Read the model definition and answer for the solid it produces. Units are mm, in the model's axes. A direction names the side the tool comes from. Round coordinates to 2 decimals unless told otherwise and drop trailing zeros. Order: outer loops, then holes, each group sorted by start corner. A loop starts at its lowest first (then second) coordinate and runs counter-clockwise, first axis right, second up. Notation, with made-up numbers: (-29.75, 56) -> (-9.75, 56) arc R25 cw to (-9.75, 85) -> close; hole circle Ø2 at (-27, 35). An arc over 180 degrees is marked (long way). One line per item, written item: value. Start each with the question number.
1. For faces 1 (the face through (0, 21, -23.5)), 2 (the face through (0, 13, 23)), 3 (the face through (0, 12, -32)), 4 (the face through (-0.063, 81.182, 64.866)), determine the directions among +Z, -Z, +X, -X, +Y, -Y from which every point of the face is accessible in a straight line to the end or side of a thin tool.
2. Section D-D (z = 10) is taken. Give the vertices of the cut face in (x, y), then the cut area to 3 significant figures.
3. The mould has two halves that part along Y. Classify faces 5 (the face through (0, 9, -37)), 6 (the face through (-11.82, -1.41, 7.9)), 7 (the face through (-0.189, 58.227, 18.773)): released by +Y, released by -Y, zero draft, split by the parting line, or undercut.
4. Section B-B (x = -1.25) is taken. Give the vertices of the cut face in (y, z).
5. Consider line 1 (Y direction, x = -12, z = 30); line 2 (X direction, y = -5, z = 17); line 3 (Z direction, x = -2.75, y = 20.5). Determine where each line is inside the solid, lowest interval first.
6. Section C-C (y = 46.8) is taken. Give the vertices of the cut face in (x, z), then the cut area to 3 significant figures.
7. Flat-ended cylindrical pins translate along their axes: pin 1 Ø5.5 at (y, z) = (-1.5, -30) entering from -X; pin 2 Ø14 at (x, y) = (-4.5, 25) entering from +Z; pin 3 Ø12 at (x, y) = (-4.5, -4.5) entering from +Z; pin 4 Ø2 at (x, y) = (1, 44) entering from -Z. Find the tip coordinate at first contact, or state that the pin passes through.
8. Section A-A (z = -30) is taken. Give the vertices of the cut face in (x, y).
from build123d import *

# Parameters (mm, degrees)
SKETCH1_W           = 27
SKETCH1_H           = 24
BOSS_EXTRUDE1_DEPTH = 37
SHELL1_T            = -3.5
BOSS_EXTRUDE2_DEPTH = 27
SHELL2_START        = -10
SHELL2_DEPTH        = 20
SKETCH3_R           = 2.1
CUT_EXTRUDE1_DEPTH  = 116.92964185
MOVE_FACE1_BY       = 0.1
MOVE_FACE1_2_BY     = 0.1
SKETCH4_R           = 2.1
CUT_EXTRUDE2_DEPTH  = 116.92964185
FILLET1_R           = 5
SKETCH5_W           = 74
SKETCH5_H           = 0.5
CUT_EXTRUDE3_DEPTH  = 116.92964185


# Read off the part's stored shape, not the designer's step: Shell2
with BuildPart() as part:
    # Sketch1 → Boss-Extrude1 (new, symmetric)
    with BuildSketch(Plane.XY):
        Rectangle(SKETCH1_W, SKETCH1_H)
    extrude(amount=BOSS_EXTRUDE1_DEPTH, both=True)

    # Shell1
    shell1_openings = [part.faces().sort_by_distance(p)[0] for p in [
        (0, 0, 37),
        (0, 0, -37),
        (0, -12, 0),
    ]]
    offset(amount=SHELL1_T, openings=shell1_openings, kind=Kind.INTERSECTION)

    # Sketch2 → Boss-Extrude2 (add)
    with BuildSketch(Plane.ZY.offset(13.5)):
        Polygon((63.282032303, 83.924355653), (-27, 31.8), (-27, 12), (21, 12), (21, 31.8), (75.282032303, 63.139745962), align=None)
    extrude(amount=-BOSS_EXTRUDE2_DEPTH)

    # Shell2 outline → Shell2 (cut)
    with BuildSketch(Plane.YZ.offset(SHELL2_START)):
        Polygon((29.779274058, 17.5), (12, 17.5), (12, -23.5), (29.779274058, -23.5), (80.89326674, 65.032032303), (63.139745962, 75.282032303), (31.8, 21), align=None)
    extrude(amount=SHELL2_DEPTH, mode=Mode.SUBTRACT)

    # Sketch3 → Cut-Extrude1 (cut, through all)
    with BuildSketch(Plane.ZY.offset(13.5)):
        with Locations((-30, -1.5)):
            Circle(SKETCH3_R)
        with Locations((-10, -1.5)):
            Circle(SKETCH3_R)
        with Locations((10, -1.5)):
            Circle(SKETCH3_R)
        with Locations((30, -1.5)):
            Circle(SKETCH3_R)
    extrude(amount=-CUT_EXTRUDE1_DEPTH, mode=Mode.SUBTRACT)

    # Move Face1: a face moved inward by 0.1
    extrude(part.faces().sort_by_distance((10, -1.759479058, 0))[0], amount=MOVE_FACE1_BY, dir=(1, 0, 0), mode=Mode.SUBTRACT)

    # Move Face1 2: a face moved inward by 0.1
    extrude(part.faces().sort_by_distance((-10, -1.759479058, 0))[0], amount=MOVE_FACE1_2_BY, dir=(-1, 0, 0), mode=Mode.SUBTRACT)

    # Sketch4 → Cut-Extrude2 (cut, through all)
    with BuildSketch(Plane.ZY.offset(13.5)):
        with Locations((61.621778265, 66.8)):
            Circle(SKETCH4_R)
        with Locations((44.301270189, 56.8)):
            Circle(SKETCH4_R)
        with Locations((26.980762114, 46.8)):
            Circle(SKETCH4_R)
    extrude(amount=-CUT_EXTRUDE2_DEPTH, mode=Mode.SUBTRACT)

    # Fillet1
    fillet1_edges = [part.edges().sort_by_distance(p)[0] for p in [
        (11.75, 31.8, 21),
        (0, 12, 21),
        (-11.75, 31.8, 21),
    ]]
    fillet(fillet1_edges, radius=FILLET1_R)

    # Sketch5 → Cut-Extrude3 (cut, through all)
    with BuildSketch(Plane.ZY.offset(13.5)):
        with Locations((0, -11.75)):
            Rectangle(SKETCH5_W, SKETCH5_H)
    extrude(amount=-CUT_EXTRUDE3_DEPTH, mode=Mode.SUBTRACT)


solid = part.part
Answer:
1. face 1: none
1. face 2: +Z, +X, -X
1. face 3: -Z, +X, -X, +Y
1. face 4: +Z, +X, -X, +Y
2. outline: (-13.5, -11.5) -> (-10.1, -11.5) -> (-10.1, -3.6) -> (-13.5, -3.6) -> close; (-13.5, 0.6) -> (-10.1, 0.6) -> (-10.1, 8.5) -> (10.1, 8.5) -> (10.1, 0.6) -> (13.5, 0.6) -> (13.5, 53.16) -> (-13.5, 53.16) -> close; (10.1, -11.5) -> (13.5, -11.5) -> (13.5, -3.6) -> (10.1, -3.6) -> close; hole (-10, 12) -> (10, 12) -> (10, 49.12) -> (-10, 49.12) -> close
2. area: 571 mm^2
3. face 5: zero draft
3. face 6: undercut
3. face 7: released by +Y
4. outline: (8.5, -37) -> (12, -37) -> (12, -27) -> (31.8, -27) -> (83.92, 63.28) -> (80.89, 65.03) -> (29.78, -23.5) -> (12, -23.5) -> (12, 17.5) -> (29.78, 17.5) -> (31.8, 21) -> (17, 21) arc R5 cw to (12, 26) -> (12, 37) -> (8.5, 37) -> close
5. line 1: -11.5 to -3.6, 0.6 to 12, 37 to 64.71
5. line 2: -13.5 to -10.1, 10.1 to 13.5
5. line 3: -27 to -23.5, 17.5 to 21
6. outline: (-13.5, -1.02) -> (13.5, -1.02) -> (13.5, 24.88) -> (10, 24.88) -> (10, 5.98) -> (-10, 5.98) -> (-10, 24.88) -> (-13.5, 24.88) -> close; (-13.5, 29.08) -> (-10, 29.08) -> (-10, 46.98) -> (-13.5, 46.98) -> close; (10, 29.08) -> (13.5, 29.08) -> (13.5, 46.98) -> (10, 46.98) -> close
6. area: 447 mm^2
7. pin 1: x = -13.5
7. pin 2: z = 21.02
7. pin 3: z = 37
7. pin 4: z = -7.6
8. outline: (-13.5, -11.5) -> (-10.1, -11.5) -> (-10.1, -3.6) -> (-13.5, -3.6) -> close; (-13.5, 0.6) -> (-10.1, 0.6) -> (-10.1, 8.5) -> (10.1, 8.5) -> (10.1, 0.6) -> (13.5, 0.6) -> (13.5, 12) -> (-13.5, 12) -> close; (10.1, -11.5) -> (13.5, -11.5) -> (13.5, -3.6) -> (10.1, -3.6) -> close
